```python
from build123d import *

# Parameters (mm, degrees)
F1_DEPTH       = 20
F2_R           = 10
F3_R           = 5
F4_R           = 5
F5_R           = 2
F6_R           = 2.5
F8_D           = 4
F8_CSINK_D     = 7
F8_CSINK_ANGLE = 90


with BuildPart() as f1:
    # F0 (on Right) → F1 (new body)
    with BuildSketch(Plane.YZ):
        Polygon((0, 60), (0, 0), (25, 0), (35.606602, 10.606602), (32.071068, 14.142136), (22.928932, 5), (5, 5), (5, 56.105373), (72.130849, 95.084579), (69.620171, 99.408524), align=None)
    extrude(amount=F1_DEPTH)

    # F2
    f2_edges = [f1.edges().sort_by_distance(p)[0] for p in [
        (10, 0, 60),
        (10, 0, 0),
        (10, 25, 0),
    ]]
    fillet(f2_edges, radius=F2_R)

    # F3
    f3_edges = [f1.edges().sort_by_distance(p)[0] for p in [
        (10, 5, 56.105373),
        (10, 5, 5),
    ]]
    fillet(f3_edges, radius=F3_R)

    # F4
    f4_edges = [f1.edges().sort_by_distance(p)[0] for p in [
        (10, 22.928932, 5),
    ]]
    fillet(f4_edges, radius=F4_R)

    # F5
    f5_edges = [f1.edges().sort_by_distance(p)[0] for p in [
        (20, 33.838835, 12.374369),
        (0, 33.838835, 12.374369),
    ]]
    fillet(f5_edges, radius=F5_R)

    # F6
    f6_edges = [f1.edges().sort_by_distance(p)[0] for p in [
        (20, 70.87551, 97.246551),
        (0, 70.87551, 97.246551),
    ]]
    fillet(f6_edges, radius=F6_R)

    # F8 (through all)
    with Locations(Plane(origin=(0, 5, 0), x_dir=(-1, 0, 0), z_dir=(0, 1, 0))):
        with Locations((-6, 30), (-14, 43.226842)):
            CounterSinkHole(F8_D / 2, F8_CSINK_D / 2, counter_sink_angle=F8_CSINK_ANGLE)


solid = f1.part
```
Check sheet for the modelled part. Datum: model origin and axes. Units: mm. A direction names the side the tool comes from. Coordinates: 2 decimals unless noted, no trailing zeros. Loops run counter-clockwise (first coordinate to the right, second up) from the corner with the lowest first, then second, coordinate; pieces in that order, holes last.
1) Release check for a two-part mould opening along Y. For faces 1 (the face through (10, 15, 0)), 2 (the face through (9.86, 28.29, 10.36)), 3 (the face through (10, 32, 7)) record: released by +Y, released by -Y, zero draft, split by the parting line, or undercut.
2) Access from +Z, -Z, +X, -X, +Y, -Y to the whole of each face (thin tool, end or side, straight path). Record for faces 4 (the face through (0.57, 33.39, 11.97)), 5 (the face through (19.399, 33.411, 11.996)), 6 (the face through (10, 16, 5)), 7 (the face through (10.14, 2.85, 3.01)), 8 (the face through (9.86, 39.358, 76.055)).
3) Sectioned sample at B-B (x = 14). Record the boundary of the cut face in (y, z).
4) Material ranges on probe 1 along X at (y, z) = (0.95, 30); probe 2 along Z at (x, y) = (14.25, 14); probe 3 along Z at (x, y) = (6, 2.35), recorded low to high.
5) Sectioned sample at A-A (z = 30). Record the boundary of the cut face in (x, y).
6) Sectioned sample at C-C (y = 29). Record the boundary of the cut face in (x, z).
7) Gauge pin test, flat ends, axial feed: pin 1 (12 mm diameter, centred on x = 4, z = 73, fed in from +Y); pin 2 (6 mm diameter, centred on x = 6.5, z = 59.5, fed in from -Y); pin 3 (1.5 mm diameter, centred on x = 16.5, y = 42.5, fed in from +Z). Record the tip position at first contact, or that the pin passes through.
8) Sectioned sample at D-D (z = 7.5). Record the boundary of the cut face in (x, y), and give its area (3 significant figures).
Check sheet entries:
1. face 1: zero draft
1. face 2: undercut
1. face 3: released by +Y
2. face 4: -X, +Y
2. face 5: +X, +Y
2. face 6: +X, -X
2. face 7: -Z, +X, -X, -Y
2. face 8: +X, -X, +Y
3. outline: (0, 10) arc R10 ccw to (10, 0) - (20.86, 0) arc R10 ccw to (27.93, 2.93) - (35.61, 10.61) - (32.07, 14.14) - (24.39, 6.46) arc R5 cw to (20.86, 5) - (10, 5) arc R5 cw to (5, 10) - (5, 39.73) - (3.5, 41.23) - (0, 41.23) - close; (0, 45.23) - (3.5, 45.23) - (5, 46.73) - (5, 53.23) arc R5 cw to (7.49, 57.55) - (72.13, 95.08) - (69.62, 99.41) - (5.07, 62.87) arc R10 ccw to (0, 54.17) - close
4. probe 1: x = 0 to 4, 8 to 20
4. probe 2: z = 0 to 5, 61.33 to 67.92
4. probe 3: z = 3.56 to 28, 32 to 60.61
5. outline: (0, 0) - (4, 0) - (4, 3.5) - (2.5, 5) - (0, 5) - close; (8, 0) - (20, 0) - (20, 5) - (9.5, 5) - (8, 3.5) - close
6. outline: (0, 4) - (20, 4) - (20, 11.07) - (0, 11.07) - close; (0, 70.04) - (20, 70.04) - (20, 76.42) - (0, 76.42) - close
7. pin 1: stops at y = 44.43
7. pin 2: stops at y = 0.28
7. pin 3: stops at z = 84.48
8. outline: (0, 0.32) - (20, 0.32) - (20, 5.67) - (0, 5.67) - close; (0, 25.43) - (20, 25.43) - (20, 32.5) - (0, 32.5) - close
8. area: 248 mm2
